Source: CAD feature listing. Evaluate the final solid. Frame: model axes, mm. Face numbers are marked on the shaded views. A direction names the side the tool comes from. Give positions to 0.01 mm unless a question says otherwise; leave off trailing zeros. Order: outer loops, then holes, each group sorted by start corner. A loop starts at its lowest first (then second) coordinate and runs counter-clockwise, first axis right, second up. Notation, with made-up numbers: M 77,58 L 103,58 A28 ccw 103,81 Z; hole C -28.75,4.5 d11. An arc over 180 degrees is marked long. Use CSV: the item, a comma, the result in double quotes. Start each with the question number.
Item 1: Ray query, probe 1 along Y at (x, z) = (-10.5, 1.65); probe 2 along Z at (x, y) = (-10.25, 21.65); probe 3 along Y at (x, z) = (-16.5, 3.5). Return the intervals inside material, ascending. Write a range as from..to.
Item 2: Section query C-C on x = -10.25. Return loops of the section in (y, z).
Item 3: Section query A-A on z = 13.5. Return loops of the section in (x, y) (3 decimals).
Item 4: Section query D-D on z = 9.75. Return loops of the section in (x, y).
Item 5: Pull-direction query (X, two-part tool) for the marked faces 6, 7 and 8; classes: +X half, -X half, draft (parallel to the pull), parting line (faces both ways), or undercut.
Item 6: First-contact query: pin 1 (8 mm diameter, centred on y = -13.5, z = 12.5, fed in from +X); pin 2 (1.5 mm diameter, centred on y = -18, z = 14, fed in from -X); pin 3 (10 mm diameter, centred on x = -9.5, y = -9.5, fed in from -Z); pin 4 (10 mm diameter, centred on x = -9.5, z = 6.5, fed in from -Y). Flat tips, straight axial feed; report the tip coordinate or a pass-through.
Item 7: Access query for the marked faces 1, 2, 3, 4 and 5. Directions: +Z, -Z, +X, -X, +Y, -Y. A direction counts if a zero-diameter tool reaches every point of the face in a straight line with its end or side. Return the directions, or none.
Item 8: Section query B-B on y = 11. Return loops of the section in (x, z), and give its area (3 significant figures).
from build123d import *

# Parameters (mm, degrees)
BOSS_EXTRUDE1_DEPTH   = 23.5
BOSS_EXTRUDE2_DEPTH   = 3
SKETCH2_W             = 20.5
SKETCH2_H             = 20.5
BOSS_EXTRUDE2_2_DEPTH = 3
SKETCH5_W             = 20.5
SKETCH5_H             = 3
BOSS_EXTRUDE4_DEPTH   = 23.5
FILLET5_R             = 3
CUT_EXTRUDE5_DEPTH    = 60.975535321
SKETCH16_R            = 2.5
CUT_EXTRUDE7_DEPTH    = 40
SKETCH17_R            = 2.5
CUT_EXTRUDE8_DEPTH    = 68.687454275
SKETCH23_R            = 2.5
CUT_EXTRUDE14_DEPTH   = 59.864801342


with BuildPart() as part:
    # Sketch1 → Boss-Extrude1 (new body)
    with BuildSketch(Plane.XY):
        Polygon((0, 0), (0, 23.5), (25, 23.5), (37.5, 1.849364905), (17.148403011, -9.900635095), (11.432268674, 0), align=None)
    extrude(amount=BOSS_EXTRUDE1_DEPTH)



with BuildPart() as body_2:
    # Sketch2 → Boss-Extrude2 (new body)
    with BuildSketch(Plane.XY):
        Polygon((17.148403011, -9.900635095), (34.901923789, 0.349364905), (45.151923789, -17.404155872), (27.398403011, -27.654155872), align=None)
    extrude(amount=BOSS_EXTRUDE2_DEPTH)


with BuildPart() as body_3:
    # Sketch2 → Boss-Extrude2 2 (new body)
    with BuildSketch(Plane.XY):
        with Locations((-10.25, 10.25)):
            Rectangle(SKETCH2_W, SKETCH2_H)
    extrude(amount=BOSS_EXTRUDE2_2_DEPTH)


with BuildPart() as part_1:
    add(part.part)

    add(body_2.part)  # Boss-Extrude4 merges body 2

    add(body_3.part)  # Boss-Extrude4 merges body 3
    # Sketch5 → Boss-Extrude4 (add)
    with BuildSketch(Plane.XY.offset(23.5)):
        with Locations((-10.25, 22)):
            Rectangle(SKETCH5_W, SKETCH5_H)
        Polygon((34.901923789, 0.349364905), (37.5, 1.849364905), (47.75, -15.904155872), (45.151923789, -17.404155872), align=None)
    extrude(amount=-BOSS_EXTRUDE4_DEPTH)

    # Fillet5
    fillet5_edges = [part_1.edges().sort_by_distance(p)[0] for p in [
        (11.432268674, 0, 11.75),
    ]]
    fillet(fillet5_edges, radius=FILLET5_R)

    # Sketch14 → Cut-Extrude5 (cut, through all)
    with BuildSketch(Plane.XY.offset(23.5)):
        Polygon((18.765371804, 23.5), (28.117314098, 18.100653599), (30.117314098, 21.564755215), (20.765371804, 26.964101615), align=None)
    extrude(amount=-CUT_EXTRUDE5_DEPTH, mode=Mode.SUBTRACT)

    # Sketch16 → Cut-Extrude7 (cut)
    with BuildSketch(Plane.XZ.offset(-20.5)):
        with Locations((-10.25, 13.5)):
            Circle(SKETCH16_R)
    extrude(amount=-CUT_EXTRUDE7_DEPTH, mode=Mode.SUBTRACT)

    # Sketch17 → Cut-Extrude8 (cut, through all)
    with BuildSketch(Plane(origin=(26.327722283, 15.200317547, 0), x_dir=(0, 0, 1), z_dir=(-0.8660254037844385, -0.5000000000000003, 0))):
        with Locations(Location((13.5, -27.398403011, 0), (0, 0, 270))):
            Circle(SKETCH17_R)
    extrude(amount=-CUT_EXTRUDE8_DEPTH, mode=Mode.SUBTRACT)

    # Sketch23 → Cut-Extrude14 (cut, through all)
    with BuildSketch(Plane.XY.offset(3)):
        with Locations((-10.5, 10)):
            Circle(SKETCH23_R)
        with Locations((31.058657049, -13.993901834)):
            Circle(SKETCH23_R)
    extrude(amount=-CUT_EXTRUDE14_DEPTH, mode=Mode.SUBTRACT)


solid = part_1.part
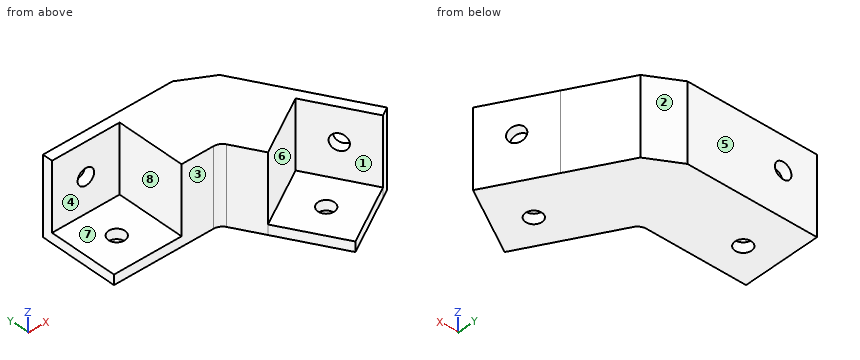
Verdict:
1,probe 1,"0..7.5, 12.5..23.5"
1,probe 2,"0..11, 16..23.5"
1,probe 3,"20.5..23.5"
2,outline,"M 0,0 L 7.51,0 L 7.51,3 L 0,3 Z; M 12.49,0 L 23.5,0 L 23.5,11 L 20.5,11 L 20.5,3 L 12.49,3 Z; M 20.5,16 L 23.5,16 L 23.5,23.5 L 20.5,23.5 Z"
3,outline,"M -20.5,20.5 L -12.75,20.5 L -12.75,23.5 L -20.5,23.5 Z; M -7.75,20.5 L 0,20.5 L 0,0 L 9.7,0 A3 cw 12.298,-1.5 L 17.148,-9.901 L 34.902,0.349 L 38.777,-6.362 L 41.375,-4.862 L 28.117,18.101 L 18.765,23.5 L -7.75,23.5 Z; M 41.277,-10.692 L 45.152,-17.404 L 47.75,-15.904 L 43.875,-9.192 Z"
4,outline,"M -20.5,20.5 L 0,20.5 L 0,0 L 9.7,0 A3 cw 12.3,-1.5 L 17.15,-9.9 L 34.9,0.35 L 45.15,-17.4 L 47.75,-15.9 L 28.12,18.1 L 18.77,23.5 L -20.5,23.5 Z"
5,face 6,"undercut"
5,face 7,"draft"
5,face 8,"-X half"
6,pin 1,"x = 47.75"
6,pin 2,"x = 45.06"
6,pin 3,"through"
6,pin 4,"y = 0"
7,face 1,"+Z, -Y"
7,face 2,"+Z, -Z, +X, +Y"
7,face 3,"+Z, -Z, -X, -Y"
7,face 4,"+Z, -X, -Y"
7,face 5,"+Z, -Z, +X, -X, +Y"
8,outline,"M -20.5,0 L -12.79,0 L -12.79,3 L -20.5,3 Z; M -8.21,0 L 32.22,0 L 32.22,23.5 L 0,23.5 L 0,3 L -8.21,3 Z"
8,area,"805 mm2"
